Can you work these out from the model? Positions are in its coordinate system, mm. A direction names the side the tool comes from. Give positions to 0.01 mm unless a question says otherwise; leave off trailing zeros. Order: outer loops, then holes, each group sorted by start corner. A loop starts at its lowest first (then second) coordinate and runs counter-clockwise, first axis right, second up. Notation, with made-up numbers: (25.25, 4) -> (71.25, 4) arc R30 ccw to (71.25, 39) -> close; hole circle Ø5 at (78.25, 77). An arc over 180 degrees is marked (long way). Answer as CSV lines item,"result".
```python
from build123d import *

# Parameters (mm, degrees)
AUFSATZ_LINEAR_AUSTRAGEN1_DEPTH      = 16
SCHNITT_LINEAR_AUSTRAGEN1_REACH      = 30.076
SKIZZE2_R                            = 1.5
SKIZZE2_R_2                          = 3
M3_GEWINDEBOHRUNG1_D                 = 2.5
M3_GEWINDEBOHRUNG1_DEPTH             = 3
M3_GEWINDEBOHRUNG1_TIP               = 0.751075774
F_1_5_1_5_DURCHMESSER_BOHRUNG1_D     = 1.5
F_1_5_1_5_DURCHMESSER_BOHRUNG1_DEPTH = 4
F_1_5_1_5_DURCHMESSER_BOHRUNG1_TIP   = 0.450645464
F_2_0_2_DURCHMESSER_BOHRUNG1_D       = 2
F_2_0_2_DURCHMESSER_BOHRUNG1_DEPTH   = 2
F_2_0_2_DURCHMESSER_BOHRUNG1_TIP     = 0.600860619
FASE1_SIZE                           = 0.5


with BuildPart() as part:
    # Skizze1 → Aufsatz-Linear austragen1 (new body)
    with BuildSketch(Plane.XY):
        with BuildLine():
            Line((-20, 4.75), (-14.43055029, 4.75))
            ThreePointArc((-14.43055029, 4.75), (-8.475, 4), (-14.43055029, 3.25))
            Line((-14.43055029, 3.25), (-20, 3.25))
            Line((-20, 3.25), (-20, 0))
            Line((-20, 0), (0, 0))
            Line((0, 0), (0, 11.5))
            Line((0, 11.5), (-20, 11.5))
            Line((-20, 11.5), (-20, 4.75))
        make_face()
    extrude(amount=AUFSATZ_LINEAR_AUSTRAGEN1_DEPTH)

    # Schnitt-Linear austragen1: up to this face of the body (flat: up to its plane)
    schnitt_linear_austragen1_end = Plane(part.part.faces().sort_by_distance((-10, 0, 8))[0])
    # Skizze2 → Schnitt-Linear austragen1 (cut, up to the picked face)
    with BuildSketch(Plane(origin=(0, 11.5, 0), x_dir=(1, 0, 0), z_dir=(0, 1, 0)), mode=Mode.PRIVATE) as schnitt_linear_austragen1_sk1:
        with Locations(Location((-17.5, -8, 0), (0, 0, 180))):
            Circle(SKIZZE2_R)
    schnitt_linear_austragen1_tool1 = split(extrude(schnitt_linear_austragen1_sk1.sketch, amount=-SCHNITT_LINEAR_AUSTRAGEN1_REACH, mode=Mode.PRIVATE), bisect_by=schnitt_linear_austragen1_end, keep=Keep.BOTH, mode=Mode.PRIVATE)
    # Skizze2 → Schnitt-Linear austragen1 (cut, up to the picked face)
    with BuildSketch(Plane(origin=(0, 11.5, 0), x_dir=(1, 0, 0), z_dir=(0, 1, 0)), mode=Mode.PRIVATE) as schnitt_linear_austragen1_sk2:
        with Locations(Location((-4.5, -8, 0), (0, 0, 180))):
            Circle(SKIZZE2_R_2)
    schnitt_linear_austragen1_tool2 = split(extrude(schnitt_linear_austragen1_sk2.sketch, amount=-SCHNITT_LINEAR_AUSTRAGEN1_REACH, mode=Mode.PRIVATE), bisect_by=schnitt_linear_austragen1_end, keep=Keep.BOTH, mode=Mode.PRIVATE)
    add(schnitt_linear_austragen1_tool1.solids().sort_by(Axis((-17.5, 11.5, 8), (0, -1, 0)))[0], mode=Mode.SUBTRACT)
    add(schnitt_linear_austragen1_tool2.solids().sort_by(Axis((-4.5, 11.5, 8), (0, -1, 0)))[0], mode=Mode.SUBTRACT)

    # M3 Gewindebohrung1
    with Locations(Plane.XY.offset(16)):
        with Locations((-3.5, 4.8)):
            Hole(M3_GEWINDEBOHRUNG1_D / 2, depth=M3_GEWINDEBOHRUNG1_DEPTH)
            with Locations((0, 0, -(M3_GEWINDEBOHRUNG1_DEPTH + M3_GEWINDEBOHRUNG1_TIP / 2))):  # 118° drill point
                Cone(0, M3_GEWINDEBOHRUNG1_D / 2, M3_GEWINDEBOHRUNG1_TIP, mode=Mode.SUBTRACT)

    # Ø1.5 (1.5) Durchmesser Bohrung1
    with Locations(Plane.XY.offset(16)):
        with Locations((-2, 2)):
            Hole(F_1_5_1_5_DURCHMESSER_BOHRUNG1_D / 2, depth=F_1_5_1_5_DURCHMESSER_BOHRUNG1_DEPTH)
            with Locations((0, 0, -(F_1_5_1_5_DURCHMESSER_BOHRUNG1_DEPTH + F_1_5_1_5_DURCHMESSER_BOHRUNG1_TIP / 2))):  # 118° drill point
                Cone(0, F_1_5_1_5_DURCHMESSER_BOHRUNG1_D / 2, F_1_5_1_5_DURCHMESSER_BOHRUNG1_TIP, mode=Mode.SUBTRACT)

    # Ø2.0 (2) Durchmesser Bohrung1
    with Locations(Plane.XY.offset(16)):
        with Locations((-2, 2)):
            Hole(F_2_0_2_DURCHMESSER_BOHRUNG1_D / 2, depth=F_2_0_2_DURCHMESSER_BOHRUNG1_DEPTH)
            with Locations((0, 0, -(F_2_0_2_DURCHMESSER_BOHRUNG1_DEPTH + F_2_0_2_DURCHMESSER_BOHRUNG1_TIP / 2))):  # 118° drill point
                Cone(0, F_2_0_2_DURCHMESSER_BOHRUNG1_D / 2, F_2_0_2_DURCHMESSER_BOHRUNG1_TIP, mode=Mode.SUBTRACT)

    # Fase1
    fase1_edges = [part.edges().sort_by_distance(p)[0] for p in [
        (-20, 8.125, 16),
        (-10, 11.5, 0),
        (0, 5.75, 0),
        (0, 0, 8),
        (-20, 0, 8),
        (-20, 11.5, 8),
        (0, 11.5, 8),
        (-20, 1.625, 16),
        (-10, 0, 16),
        (0, 5.75, 16),
        (-10, 11.5, 16),
        (-10, 0, 0),
        (-20, 1.625, 0),
        (-20, 8.125, 0),
    ]]
    chamfer(fase1_edges, length=FASE1_SIZE)


solid = part.part
```
Item 1: Please list where these lines run through material, in increasing order: line 1 along Y through (x, z) = (-11.5, 4) (3 decimals); line 2 along X through (y, z) = (5.5, 7); line 3 along X through (y, z) = (4.8, 14.2).
Numbers:
line 1,"y = 0 to 0.975, 7.025 to 11.5"
line 2,"x = -20 to -18.62, -16.38 to -14.13, -8.87 to -7.33, -1.67 to 0"
line 3,"x = -20 to -14.42, -8.58 to -4.75, -2.25 to 0"
Item 2: Imagine slicing it at C-C, the plane y = 9. Please give me the cut outline in (x, z).
Numbers:
outline,"(-20, 0.5) -> (-19.5, 0) -> (-0.5, 0) -> (0, 0.5) -> (0, 15.5) -> (-0.5, 16) -> (-19.5, 16) -> (-20, 15.5) -> close; hole circle Ø3 at (-17.5, 8); hole circle Ø6 at (-4.5, 8)"
Item 3: For pin 1 (2.5 mm diameter, centred on x = -17.5, z = 8, fed in from +Y); pin 2 (1.5 mm diameter, centred on x = -3.5, y = 4.8, fed in from +Z), each with a flat end and sliding along its axis, tell me the tip position at first contact or that it passes through.
Numbers:
pin 1,"passes through"
pin 2,"stops at z = 12.7"
Item 4: Imagine slicing it at A-A, the plane z = 8. Please give me the cut outline in (x, y) (3 decimals), then the cut area to 3 significant figures.
Numbers:
outline,"(-20, 0.5) -> (-19.5, 0) -> (-19, 0) -> (-19, 3.25) -> (-20, 3.25) -> close; (-20, 4.75) -> (-19, 4.75) -> (-19, 11.5) -> (-19.5, 11.5) -> (-20, 11) -> close; (-16, 0) -> (-7.5, 0) -> (-7.5, 11.5) -> (-16, 11.5) -> (-16, 4.75) -> (-14.431, 4.75) arc R3.025 cw (long way) to (-14.431, 3.25) -> (-16, 3.25) -> close; (-1.5, 0) -> (-0.5, 0) -> (0, 0.5) -> (0, 11) -> (-0.5, 11.5) -> (-1.5, 11.5) -> close"
area,"93.5 mm²"
Item 5: Imagine slicing it at B-B, the plane z = 14.25. Please give me the cut outline in (x, y) (3 decimals).
Numbers:
outline,"(-20, 0.5) -> (-19.5, 0) -> (-0.5, 0) -> (0, 0.5) -> (0, 11) -> (-0.5, 11.5) -> (-19.5, 11.5) -> (-20, 11) -> (-20, 4.75) -> (-14.431, 4.75) arc R3.025 cw (long way) to (-14.431, 3.25) -> (-20, 3.25) -> close; hole circle Ø2.5 at (-3.5, 4.8); hole circle Ø2 at (-2, 2)"
Item 6: We'd pull the mould along X, two halves only. Please class faces 4 (the flat face through (-10, 7, 16)), 5 (the cylindrical face through (-4.69, 5.18, 14.48)), 6 (the flat face through (-20, 2, 8)): released by +X, released by -X, zero draft, split by the parting line, or undercut.
Numbers:
face 4,"zero draft"
face 5,"undercut"
face 6,"released by -X"
Item 7: Imagine slicing it at D-D, the plane x = -7.25. Please give me the cut outline in (y, z), then the cut area to 3 significant figures.
Numbers:
outline,"(0, 0.5) -> (0.5, 0) -> (11, 0) -> (11.5, 0.5) -> (11.5, 6.8) -> (0, 6.8) -> close; (0, 9.2) -> (11.5, 9.2) -> (11.5, 15.5) -> (11, 16) -> (0.5, 16) -> (0, 15.5) -> close"
area,"156 mm²"
Item 8: For faces 1 (the flat face through (-17, 3.25, 10)), 2 (the cylindrical face through (-2.715, 2.225, 12.912)), 3 (the cylindrical face through (-16, 2, 8)), which set-ups out of +Z, -Z, +X, -X, +Y, -Y let a thin tool reach every point of the face, with its end or its side?
Numbers:
face 1,"+Z, -Z, -X"
face 2,"+Z"
face 3,"+Y, -Y"
